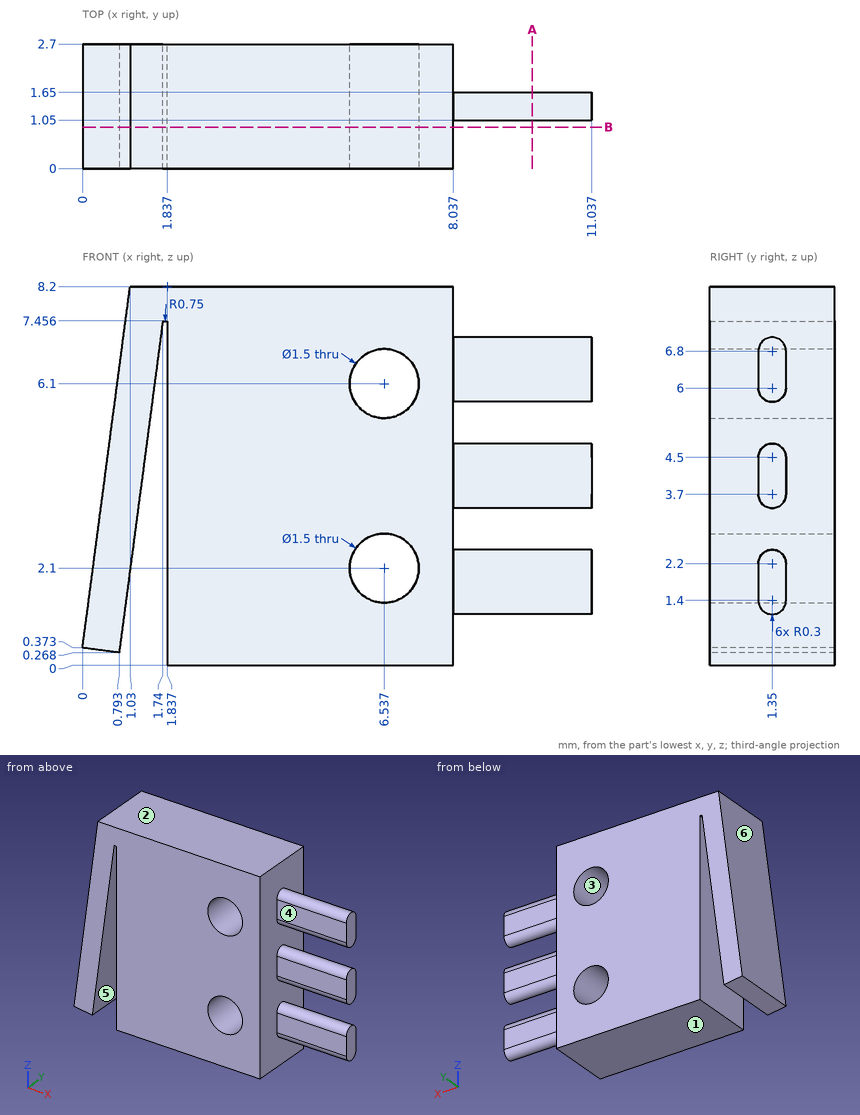
Design review of the part shown in the three views and the two pictorial views. Dimensions are in mm from the part's minimum x, y and z. A direction names the side the tool comes from. Coordinates: 2 decimals unless noted, no trailing zeros. Order: outer loops, then holes, each group sorted by start corner. A loop starts at its lowest first (then second) coordinate and runs counter-clockwise, first axis right, second up. Notation, with made-up numbers: (85.5, -8) -> (112.5, -8) arc R21 ccw to (112.5, 8) -> close; hole circle Ø2 at (55, 34). An arc over 180 degrees is marked (long way). Use one line per item in the form item = value. Start each with the question number.
(1) Add section A-A on x = 9.75. State the section outline as (y, z) points.
(2) For probe 1 along X at (y, z) = (0.45, 2) (1 decimal); probe 2 along X at (y, z) = (0.4, 1.75) (1 decimal); probe 3 along Z at (x, y) = (7, 1.6), list the stretches that pass through material, from the lowest coordinate up.
(3) The part is to be moulded in two halves that separate along Z. For the marked faces 1, 2 and 3, say which applies: +Z half, -Z half, draft (parallel to the pull), parting line (faces both ways), or undercut.
(4) Add section B-B on y = 0.9. State the section outline as (x, z) points.
(5) For the marked faces 4, 5 and 6, list the 3-axis set-ups (+Z, -Z, +X, -X, +Y, -Y) from which the entire face can be reached by the end or side of a thin tool; tool diameter is ignored.
(6) Insertion check: pin 1 (2.5 mm diameter, centred on x = 6.54, z = 6.1, fed in from +Y); pin 2 (0.6 mm diameter, centred on x = 9, z = 6.5, fed in from +Y); pin 3 (1 mm diameter, centred on y = 1, z = 6.5, fed in from -X); pin 4 (0.8 mm diameter, centred on y = 1.5, z = 4.5, fed in from -X). Each pin has a flat end and moves straight along its axis. Give the tip position at first contact, or say it passes through.
Answer block:
q1.outline = (1.05, 1.4) arc R0.3 ccw to (1.65, 1.4) -> (1.65, 2.2) arc R0.3 ccw to (1.05, 2.2) -> close; (1.05, 3.7) arc R0.3 ccw to (1.65, 3.7) -> (1.65, 4.5) arc R0.3 ccw to (1.05, 4.5) -> close; (1.05, 6) arc R0.3 ccw to (1.65, 6) -> (1.65, 6.8) arc R0.3 ccw to (1.05, 6.8) -> close
q2.probe_1 = 0.2 to 1, 1.8 to 5.8, 7.3 to 8
q2.probe_2 = 0.2 to 1, 1.8 to 5.9, 7.2 to 8
q2.probe_3 = 0 to 1.51, 2.69 to 5.51, 6.69 to 8.2
q3.face_1 = -Z half
q3.face_2 = +Z half
q3.face_3 = undercut
q4.outline = (0, 0.37) -> (0.79, 0.27) -> (1.74, 7.46) arc R0.75 ccw to (1.84, 7.45) -> (1.84, 0) -> (8.04, 0) -> (8.04, 8.2) -> (1.03, 8.2) -> close; hole circle Ø1.5 at (6.54, 2.1); hole circle Ø1.5 at (6.54, 6.1)
q5.face_4 = +Z, -Z, +X, -Y
q5.face_5 = -Z, +Y, -Y
q5.face_6 = +Z, -X, +Y, -Y
q6.pin_1 = 2.7
q6.pin_2 = 1.65
q6.pin_3 = 0.74
q6.pin_4 = 0.49
